Source: CAD feature listing. Evaluate the final solid. Frame: model axes, mm. Face numbers are marked on the shaded views. Give positions to 0.01 mm unless a question says otherwise; leave off trailing zeros. Loops run counter-clockwise (first coordinate to the right, second up) from the corner with the lowest first, then second, coordinate; pieces in that order, holes last. Notation, with made-up numbers: (-20, 60) -> (23, 60) arc R6 ccw to (23, 67) -> close; hole circle Ø3 at (66, -16.5). An arc over 180 degrees is marked (long way). Put each result on its own line as item: value.
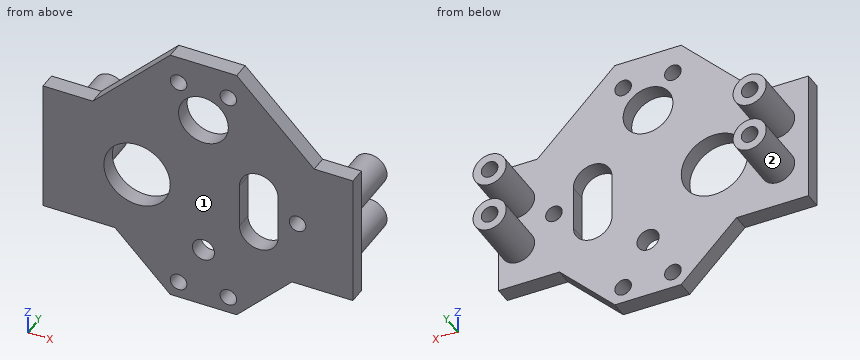
```python
from build123d import *

# Parameters (mm, degrees)
SKETCH1_W           = 12
SKETCH1_H           = 10
SKETCH1_H_2         = 24
SKETCH1_H_3         = 14
BOSS_EXTRUDE1_DEPTH = 3
SKETCH2_R           = 1.5
SKETCH2_R_2         = 2
SKETCH2_R_3         = 4.5
CUT_EXTRUDE1_DEPTH  = 3
SKETCH3_R           = 3
BOSS_EXTRUDE2_DEPTH = 10
SKETCH4_R           = 1.5
SKETCH4_R_2         = 6
CUT_EXTRUDE2_DEPTH  = 4
SKETCH5_R           = 1.5
CUT_EXTRUDE3_DEPTH  = 10


with BuildPart() as part:
    # Sketch1 → Boss-Extrude1 (new body)
    with BuildSketch(Plane(origin=(0, 0, 0), x_dir=(1, 0, 0), z_dir=(0, 1, 0))):
        Polygon((0, 0), (0, 14), (-14, 14), align=None)
        Polygon((0, 38), (-10, 38), (-23, 38), (-23, 14), (-14, 14), (0, 14), align=None)
        Polygon((22, 38), (12, 48), (12, 38), align=None)
        with Locations((6, 43)):
            Rectangle(SKETCH1_W, SKETCH1_H)
        with Locations((6, 26)):
            Rectangle(SKETCH1_W, SKETCH1_H_2)
        Polygon((22, 38), (12, 38), (12, 14), (26, 14), (33, 14), (33, 38), align=None)
        Polygon((26, 14), (12, 14), (12, 0), align=None)
        with Locations((6, 7)):
            Rectangle(SKETCH1_W, SKETCH1_H_3)
        Polygon((0, 38), (0, 48), (-10, 38), align=None)
    extrude(amount=BOSS_EXTRUDE1_DEPTH)

    # Sketch2 → Cut-Extrude1 (cut)
    with BuildSketch(Plane(origin=(0, 3, 0), x_dir=(1, 0, 0), z_dir=(0, 1, 0))):
        with Locations((1.5, 45)):
            Circle(SKETCH2_R)
        with Locations((10.5, 45)):
            Circle(SKETCH2_R)
        with Locations((10.5, 5)):
            Circle(SKETCH2_R)
        with Locations((1.5, 5)):
            Circle(SKETCH2_R)
        with Locations((6, 37)):
            Circle(SKETCH2_R_2)
        with Locations((6, 11)):
            Circle(SKETCH2_R_3)
    extrude(amount=-CUT_EXTRUDE1_DEPTH, mode=Mode.SUBTRACT)

    # Sketch3 → Boss-Extrude2 (add)
    with BuildSketch(Plane(origin=(0, 3, 0), x_dir=(1, 0, 0), z_dir=(0, 1, 0))):
        with Locations((-17.5, 30.5)):
            Circle(SKETCH3_R)
        with Locations((-17.5, 21.5)):
            Circle(SKETCH3_R)
        with Locations((29.5, 30.5)):
            Circle(SKETCH3_R)
        with Locations((29.5, 21.5)):
            Circle(SKETCH3_R)
    extrude(amount=BOSS_EXTRUDE2_DEPTH)

    # Sketch4 → Cut-Extrude2 (cut, through all)
    with BuildSketch(Plane(origin=(0, 3, 0), x_dir=(1, 0, 0), z_dir=(0, 1, 0))):
        with Locations((23, 26)):
            Circle(SKETCH4_R)
        with Locations((-6, 26)):
            Circle(SKETCH4_R_2)
        with BuildLine():
            Line((12.5, 22), (12.5, 30))
            ThreePointArc((12.5, 30), (16, 33.5), (19.5, 30))
            Line((19.5, 30), (19.5, 22))
            ThreePointArc((19.5, 22), (16, 18.5), (12.5, 22))
        make_face()
    extrude(amount=-CUT_EXTRUDE2_DEPTH, mode=Mode.SUBTRACT)

    # Sketch5 → Cut-Extrude3 (cut)
    with BuildSketch(Plane(origin=(0, 13, 0), x_dir=(1, 0, 0), z_dir=(0, 1, 0))):
        with Locations((29.5, 30.5)):
            Circle(SKETCH5_R)
        with Locations((29.5, 21.5)):
            Circle(SKETCH5_R)
        with Locations((-17.5, 30.5)):
            Circle(SKETCH5_R)
        with Locations((-17.5, 21.5)):
            Circle(SKETCH5_R)
    extrude(amount=-CUT_EXTRUDE3_DEPTH, mode=Mode.SUBTRACT)


solid = part.part
```
(1) Section A-A on y = 11.25. Return loops of the section in (x, z), then the cut area to 3 significant figures.
Calculated:
outline: circle Ø6 at (-17.5, -30.5); circle Ø6 at (-17.5, -21.5); circle Ø6 at (29.5, -30.5); circle Ø6 at (29.5, -21.5); hole circle Ø3 at (-17.5, -30.5); hole circle Ø3 at (-17.5, -21.5); hole circle Ø3 at (29.5, -30.5); hole circle Ø3 at (29.5, -21.5)
area: 84.8 mm²
(2) Section B-B on z = -45. Return loops of the section in (x, y).
Calculated:
outline: (-3, 0) -> (0, 0) -> (0, 3) -> (-3, 3) -> close; (3, 0) -> (9, 0) -> (9, 3) -> (3, 3) -> close; (12, 0) -> (15, 0) -> (15, 3) -> (12, 3) -> close
(3) Section C-C on x = 23. Return loops of the section in (y, z).
Calculated:
outline: (0, -38) -> (3, -38) -> (3, -27.5) -> (0, -27.5) -> close; (0, -24.5) -> (3, -24.5) -> (3, -11) -> (0, -11) -> close
(4) Line query: probe 1 along Z at (x, y) = (-17.5, 11.25); probe 2 along X at (y, z) = (2.25, -26); probe 3 along X at (y, z) = (5.25, -21.5). Output: solid intervals per line, ascending. Write a range as from..to.
Calculated:
probe 1: z = -33.5..-32, -29..-27.5, -24.5..-23, -20..-18.5
probe 2: x = -23..-12, 0..12.5, 19.5..21.5, 24.5..33
probe 3: x = -20.5..-19, -16..-14.5, 26.5..28, 31..32.5
(5) Section D-D on z = -26. Return loops of the section in (x, y), then the cut area to 3 significant figures.
Calculated:
outline: (-23, 0) -> (-12, 0) -> (-12, 3) -> (-23, 3) -> close; (0, 0) -> (12.5, 0) -> (12.5, 3) -> (0, 3) -> close; (19.5, 0) -> (21.5, 0) -> (21.5, 3) -> (19.5, 3) -> close; (24.5, 0) -> (33, 0) -> (33, 3) -> (24.5, 3) -> close
area: 102 mm²
(6) First-contact query: P1, Ø5, axis at x = -5, y = 3, coming from the +Z side; P2, Ø12, axis at x = -15, z = -41, coming from the +Y side; P3, Ø6, axis at x = 24, y = 11.5, coming from the -Z side. Flat tips, straight axial feed; report the tip coordinate or a pass-through.
Calculated:
P1: stops at z = -2.5
P2: stops at y = 3
P3: stops at z = -32.16
(7) Draft query along Z for the marked faces 1 and 2. Return one class per face: released by +Z, released by -Z, zero draft, split by the parting line, or undercut.
Calculated:
face 1: zero draft
face 2: undercut
